from build123d import *

# Parameters (mm, degrees)
SKETCH2_W                = 16
SKETCH2_H                = 19
BOSS_EXTRUDE1_DEPTH      = 13.3
SKETCH3_W                = 12
SKETCH3_H                = 19
CUT_EXTRUDE1_DEPTH       = 8.9
CUT_EXTRUDE2_DEPTH       = 19.19725254
CUT_EXTRUDE2_DEPTH_BACK  = 19.19725254
SKETCH4_W                = 9.9
SKETCH4_H                = 3.9
SKETCH6_W                = 14
SKETCH6_H                = 9.1
BOSS_EXTRUDE2_DEPTH      = 2.5
CUT_EXTRUDE4_DEPTH       = 21.072119968
CUT_EXTRUDE4_DEPTH_BACK  = 21.072119968
SKETCH7_R                = 1.55
BOSS_EXTRUDE3_DEPTH      = 9.5
BOSS_EXTRUDE3_DEPTH_BACK = 9.1
SKETCH14_W               = 12
SKETCH14_H               = 8.9
CUT_EXTRUDE9_DEPTH       = 22.520687721
CUT_EXTRUDE9_DEPTH_BACK  = 22.520687721
FILLET4_R                = 0.9
SKETCH16_W               = 16.145602647
SKETCH16_H               = 8.9
CUT_EXTRUDE10_DEPTH      = 9.1
SKETCH17_W               = 7
SKETCH17_H               = 2.4
BOSS_EXTRUDE4_DEPTH      = 3
FILLET6_R                = 0.5
FILLET7_R                = 0.5
FILLET8_R                = 0.5


with BuildPart() as part:
    # Sketch2 → Boss-Extrude1 (new body)
    with BuildSketch(Plane(origin=(0, 0, 0), x_dir=(1, 0, 0), z_dir=(0, 1, 0))):
        Rectangle(SKETCH2_W, SKETCH2_H)
    extrude(amount=BOSS_EXTRUDE1_DEPTH)

    # Sketch3 → Cut-Extrude1 (cut)
    with BuildSketch(Plane(origin=(0, 13.3, 0), x_dir=(1, 0, 0), z_dir=(0, 1, 0))):
        Rectangle(SKETCH3_W, SKETCH3_H)
    extrude(amount=-CUT_EXTRUDE1_DEPTH, mode=Mode.SUBTRACT)

    # Sketch4 → Cut-Extrude2 (cut, two sides: drawn at the far end of the back side and taken through both)
    with BuildSketch(Plane(origin=(0, 0, 0), x_dir=(0, 0, -1), z_dir=(1, 0, 0)).offset(-CUT_EXTRUDE2_DEPTH_BACK)):
        with Locations((-4.55, 11.35)):
            Rectangle(SKETCH4_W, SKETCH4_H)
    extrude(amount=CUT_EXTRUDE2_DEPTH + CUT_EXTRUDE2_DEPTH_BACK, mode=Mode.SUBTRACT)

    # Sketch6 → Boss-Extrude2 (add)
    with BuildSketch(Plane(origin=(0, 0, 0), x_dir=(1, 0, 0), z_dir=(0, 1, 0))):
        with Locations((7, 4.95)):
            Rectangle(SKETCH6_W, SKETCH6_H)
        with Locations((-7, 4.95)):
            Rectangle(SKETCH6_W, SKETCH6_H)
    extrude(amount=BOSS_EXTRUDE2_DEPTH)

    # Sketch7 → Cut-Extrude4 (cut, two sides: drawn at the far end of the back side and taken through both)
    with BuildSketch(Plane(origin=(0, 2.5, 0), x_dir=(1, 0, 0), z_dir=(0, 1, 0)).offset(-CUT_EXTRUDE4_DEPTH_BACK)):
        with Locations(Location((-11, 5, 0), (0, 0, 270))):
            Circle(SKETCH7_R)
        with Locations(Location((11, 5, 0), (0, 0, 270))):
            Circle(SKETCH7_R)
    extrude(amount=CUT_EXTRUDE4_DEPTH + CUT_EXTRUDE4_DEPTH_BACK, mode=Mode.SUBTRACT)

    # Sketch14 → Boss-Extrude3 (add, two sides: drawn at the far end of the back side and taken through both)
    with BuildSketch(Plane.XY.offset(-BOSS_EXTRUDE3_DEPTH_BACK)):
        with Locations((0, 8.85)):
            Rectangle(SKETCH14_W, SKETCH14_H)
    extrude(amount=BOSS_EXTRUDE3_DEPTH + BOSS_EXTRUDE3_DEPTH_BACK)

    # Sketch15 → Cut-Extrude9 (cut, two sides: drawn at the far end of the back side and taken through both)
    with BuildSketch(Plane.XY.offset(-CUT_EXTRUDE9_DEPTH_BACK)):
        with BuildLine():
            ThreePointArc((-6, 8.3), (-5.132040834, 6.102704612), (-3.494281042, 4.4))
            Line((-3.494281042, 4.4), (3.494281042, 4.4))
            ThreePointArc((3.494281042, 4.4), (5.132040834, 6.102704612), (6, 8.3))
            Line((6, 8.3), (6, 13.3))
            Line((6, 13.3), (-6, 13.3))
            Line((-6, 13.3), (-6, 8.3))
        make_face()
    extrude(amount=CUT_EXTRUDE9_DEPTH + CUT_EXTRUDE9_DEPTH_BACK, mode=Mode.SUBTRACT)

    # Fillet4
    fillet4_edges = [part.edges().sort_by_distance(p)[0] for p in [
        (-6, 4.4, -9.3),
        (6, 4.4, -9.3),
    ]]
    fillet(fillet4_edges, radius=FILLET4_R)

    # Sketch16 → Cut-Extrude10 (cut)
    with BuildSketch(Plane(origin=(0, 0, -9.5), x_dir=(-1, 0, 0), z_dir=(0, 0, -1))):
        with Locations((-0.072801324, 8.85)):
            Rectangle(SKETCH16_W, SKETCH16_H)
    extrude(amount=-CUT_EXTRUDE10_DEPTH, mode=Mode.SUBTRACT)

    # Sketch17 → Boss-Extrude4 (add)
    with BuildSketch(Plane(origin=(0, 4.4, 0), x_dir=(1, 0, 0), z_dir=(0, 1, 0))):
        with Locations((-2.5, 2.5)):
            Rectangle(SKETCH17_W, SKETCH17_H)
    extrude(amount=BOSS_EXTRUDE4_DEPTH)

    # Fillet6
    fillet6_edges = [part.edges().sort_by_distance(p)[0] for p in [
        (-2.5, 7.4, -3.7),
    ]]
    fillet(fillet6_edges, radius=FILLET6_R)

    # Fillet7
    fillet7_edges = [part.edges().sort_by_distance(p)[0] for p in [
        (-2.5, 7.4, -1.3),
    ]]
    fillet(fillet7_edges, radius=FILLET7_R)

    # Fillet8
    fillet8_edges = [part.edges().sort_by_distance(p)[0] for p in [
        (8, 4.4, -4.95),
        (-8, 4.4, -4.95),
    ]]
    fillet(fillet8_edges, radius=FILLET8_R)


solid = part.part
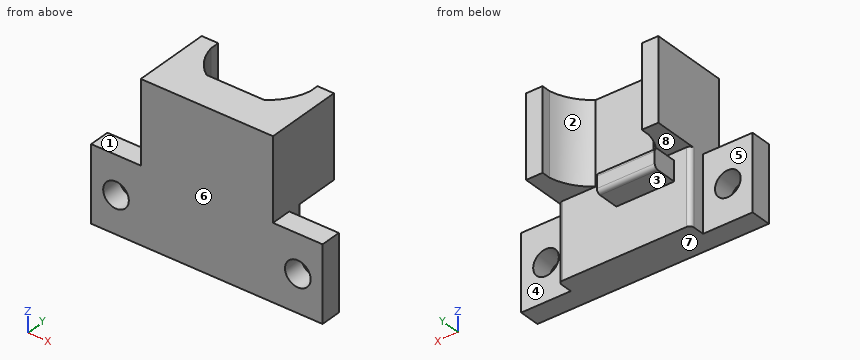
The model under review builds one solid part; all positions refer to its coordinate system, in mm. Face numbers are marked on the shaded views. A direction names the side the tool comes from. Coordinates: 2 decimals unless noted, no trailing zeros. Loops run counter-clockwise (first coordinate to the right, second up) from the corner with the lowest first, then second, coordinate; pieces in that order, holes last. Notation, with made-up numbers: (-36, -8) -> (-25, -8) arc R18 cw to (-25, 9) -> close; hole circle Ø8 at (77.5, 54). An arc over 180 degrees is marked (long way). Use a Markdown table: item, result. Add a question column.
1. Add section B-B on x = 11. Write out the cut boundary in (y, z), plus the area to 3 significant figures.
2. Machinability: for the marked faces 1, 2, 3, 4 and 5, which of the approach directions +Z, -Z, +X, -X, +Y, -Y give a long, thin tool a straight path to every point of the face, cutting with its end or side? Answer none if there is none.
3. Add section A-A on z = -5. Write out the cut boundary in (x, y).
4. Add section C-C on y = 5.5. Write out the cut boundary in (x, z).
5. Clearance check with flat-ended pins moving along their axes: pin 1 Ø0.9 at (y, z) = (9, 5.5) entering from -X; pin 2 Ø5 at (x, z) = (-4, -1.5) entering from +Y; pin 3 Ø1.2 at (x, y) = (-2, 6) entering from -Z; pin 4 Ø3 at (x, y) = (-2.5, 6) entering from +Z. State where each tip first meets the part, or that it passes through.
6. Add section D-D on z = 1. Write out the cut boundary in (x, y), plus the area to 3 significant figures.
7. To check wall thickness, follow line 1 (X direction, y = 1.85, z = -5); line 2 (Z direction, x = -11, y = 1.55); line 3 (Y direction, x = 4.25, z = -3). State the ranges of each line that lie inside material, in increasing order.
8. Draft analysis for pull direction Z (two halves, no side actions). For the marked faces 6, 7 and 8, state which applies: pulls with the +Z half, pulls with the -Z half, needs draft (parallel to the pull), parting line crosses it, or undercut.
Returned:
| question | item | result |
|---|---|---|
| 1 | outline | (0, -9.5) -> (2.5, -9.5) -> (2.5, -6.55) -> (0, -6.55) -> close; (0, -3.45) -> (2.5, -3.45) -> (2.5, -0.4) -> (0, -0.4) -> close |
| 1 | area | 15.0 mm² |
| 2 | face 1 | +Z, -X, +Y, -Y |
| 2 | face 2 | +Z, -Z, +Y |
| 2 | face 3 | -Z, +X, -X, +Y |
| 2 | face 4 | +Z, -Z, +X, +Y |
| 2 | face 5 | +Z, -Z, -X, +Y |
| 3 | outline | (-14, 0) -> (-12.55, 0) -> (-12.55, 2.5) -> (-14, 2.5) -> close; (-9.45, 0) -> (9.45, 0) -> (9.45, 2.5) -> (8, 2.5) -> (8, 3.9) arc R0.5 ccw to (7.5, 4.4) -> (-7.5, 4.4) arc R0.5 ccw to (-8, 3.9) -> (-8, 2.5) -> (-9.45, 2.5) -> close; (12.55, 0) -> (14, 0) -> (14, 2.5) -> (12.55, 2.5) -> close |
| 4 | outline | (-8, -0.4) -> (-4.69, -0.4) -> (-4.69, 9.5) -> (-8, 9.5) -> close; (-6, -3.7) -> (1, -3.7) -> (1, -1.3) -> (-6, -1.3) -> close; (4.69, -0.4) -> (8, -0.4) -> (8, 9.5) -> (4.69, 9.5) -> close |
| 5 | pin 1 | stops at x = -8 |
| 5 | pin 2 | stops at y = 9.4 |
| 5 | pin 3 | stops at z = -3.7 |
| 5 | pin 4 | stops at z = -1.3 |
| 6 | outline | (-8, 0) -> (8, 0) -> (8, 9.4) -> (6, 9.4) -> (6, 8.3) arc R6.1 cw to (3.49, 4.4) -> (-3.49, 4.4) arc R6.1 cw to (-6, 8.3) -> (-6, 9.4) -> (-8, 9.4) -> close |
| 6 | area | 97.3 mm² |
| 7 | line 1 | x = -14 to -12.55, -9.45 to 9.45, 12.55 to 14 |
| 7 | line 2 | z = -9.5 to -6.55, -3.45 to -0.4 |
| 7 | line 3 | y = 0 to 4.4 |
| 8 | face 6 | needs draft |
| 8 | face 7 | pulls with the -Z half |
| 8 | face 8 | undercut |
